Check sheet for the modelled part. Datum: model origin and axes. Units: mm. Coordinates: 2 decimals unless noted, no trailing zeros. Order: outer loops, then holes, each group sorted by start corner. A loop starts at its lowest first (then second) coordinate and runs counter-clockwise, first axis right, second up.
1. Gauge pin test, flat ends, axial feed: pin 1 Ø1 at (y, z) = (-16, 3) entering from +X; pin 2 Ø2.5 at (x, y) = (11.075, -27) entering from -Z; pin 3 Ø1.7 at (x, y) = (15.575, 21.5) entering from +Z. Record the tip position at first contact, or that the pin passes through.
2. Cross-section at C-C (y = -27). Enter the section's corners in (x, z) (3 decimals), then the cut area to 3 significant figures.
3. Thickness scan on line 1 (Y direction, x = -8.94, z = 2.9); line 2 (Y direction, x = -8.94, z = 1.95); line 3 (Y direction, x = -9.5, z = 3.3). Record the ranges inside material, lowest first.
4. Cross-section at D-D (y = -10). Enter the section's corners in (x, z) (3 decimals), then the cut area to 3 significant figures.
5. Cross-section at B-B (x = 0). Enter the section's corners in (y, z).
6. Cross-section at A-A (z = 3.4). Enter the section's corners in (x, y), then the cut area to 3 significant figures.
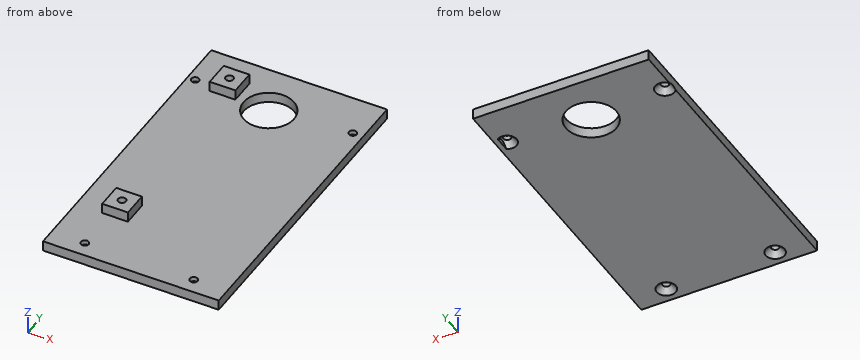
```python
from build123d import *

# Parameters (mm, degrees)
SKETCH1_W           = 33.15
SKETCH1_H           = 60
SKETCH1_R           = 4.9
BOSS_EXTRUDE1_DEPTH = 2
SKETCH3_W           = 5
SKETCH3_H           = 5
BOSS_EXTRUDE2_DEPTH = 2
SKETCH4_R           = 0.75
CUT_EXTRUDE1_DEPTH  = 2
CHAMFER1_SIZE       = 1.1
SKETCH5_W           = 2
SKETCH5_H           = 60
BOSS_EXTRUDE3_DEPTH = 1
SKETCH7_R           = 0.762
CUT_EXTRUDE2_DEPTH  = 3.5


with BuildPart() as part:
    # Sketch1 → Boss-Extrude1 (new body)
    with BuildSketch(Plane.XY):
        Rectangle(SKETCH1_W, SKETCH1_H)
        with Locations((0, 20.1)):
            Circle(SKETCH1_R, mode=Mode.SUBTRACT)
    extrude(amount=BOSS_EXTRUDE1_DEPTH)

    # Sketch3 → Boss-Extrude2 (add)
    with BuildSketch(Plane.XY.offset(2)):
        with Locations((-8.94, 22.5)):
            Rectangle(SKETCH3_W, SKETCH3_H)
        with Locations((-8.94, -15.82)):
            Rectangle(SKETCH3_W, SKETCH3_H)
    extrude(amount=BOSS_EXTRUDE2_DEPTH)

    # Sketch4 → Cut-Extrude1 (cut)
    with BuildSketch(Plane(origin=(0, 0, 0), x_dir=(-1, 0, 0), z_dir=(0, 0, -1))):
        with Locations((-15.575, 21.5)):
            Circle(SKETCH4_R)
        with Locations((15.075, 21.5)):
            Circle(SKETCH4_R)
        with Locations((10.075, -27)):
            Circle(SKETCH4_R)
        with Locations((-11.075, -27)):
            Circle(SKETCH4_R)
    extrude(amount=-CUT_EXTRUDE1_DEPTH, mode=Mode.SUBTRACT)

    # Chamfer1
    # the kernel refuses this chamfer: 1.1 mm, written as the material it takes off along each edge
    with BuildSketch(Plane(origin=(15.575, 21.5, 0), x_dir=(-1, 0, 0), z_dir=(0, -1, 0))) as chamfer1_piece_1:
        Polygon((0.75 + CHAMFER1_SIZE, 0), (0.75, -CHAMFER1_SIZE), (0.75, 0), align=None)
    revolve(axis=Axis((15.575, 21.5, 0), (0, 0, -1)), mode=Mode.SUBTRACT)
    with BuildSketch(Plane(origin=(-15.075, 21.5, 0), x_dir=(-1, 0, 0), z_dir=(0, -1, 0))) as chamfer1_piece_2:
        Polygon((0.75 + CHAMFER1_SIZE, 0), (0.75, -CHAMFER1_SIZE), (0.75, 0), align=None)
    revolve(axis=Axis((-15.075, 21.5, 0), (0, 0, -1)), mode=Mode.SUBTRACT)
    with BuildSketch(Plane(origin=(-10.075, -27, 0), x_dir=(-1, 0, 0), z_dir=(0, -1, 0))) as chamfer1_piece_3:
        Polygon((0.75 + CHAMFER1_SIZE, 0), (0.75, -CHAMFER1_SIZE), (0.75, 0), align=None)
    revolve(axis=Axis((-10.075, -27, 0), (0, 0, -1)), mode=Mode.SUBTRACT)
    with BuildSketch(Plane(origin=(11.075, -27, 0), x_dir=(-1, 0, 0), z_dir=(0, -1, 0))) as chamfer1_piece_4:
        Polygon((0.75 + CHAMFER1_SIZE, 0), (0.75, -CHAMFER1_SIZE), (0.75, 0), align=None)
    revolve(axis=Axis((11.075, -27, 0), (0, 0, -1)), mode=Mode.SUBTRACT)

    # Sketch5 → Boss-Extrude3 (add)
    with BuildSketch(Plane(origin=(16.575, 0, 0), x_dir=(0, 0, -1), z_dir=(1, 0, 0))):
        with Locations((-1, 0)):
            Rectangle(SKETCH5_W, SKETCH5_H)
    extrude(amount=BOSS_EXTRUDE3_DEPTH)

    # Sketch7 → Cut-Extrude2 (cut)
    with BuildSketch(Plane.XY.offset(4)):
        with Locations((-8.94, 22.5)):
            Circle(SKETCH7_R)
        with Locations((-8.94, -15.82)):
            Circle(SKETCH7_R)
    extrude(amount=-CUT_EXTRUDE2_DEPTH, mode=Mode.SUBTRACT)


solid = part.part
```
Data:
1. pin 1: stops at x = -6.44
1. pin 2: stops at z = 0.6
1. pin 3: stops at z = 2
2. outline: (-16.575, 0) - (-11.925, 0) - (-10.825, 1.1) - (-10.825, 2) - (-16.575, 2) - close; (-9.325, 1.1) - (-8.225, 0) - (9.225, 0) - (10.325, 1.1) - (10.325, 2) - (-9.325, 2) - close; (11.825, 1.1) - (12.925, 0) - (17.575, 0) - (17.575, 2) - (11.825, 2) - close
2. area: 59.9 mm2
3. line 1: y = -18.32 to -16.58, -15.06 to -13.32, 20 to 21.74, 23.26 to 25
3. line 2: y = -30 to -16.58, -15.06 to 21.74, 23.26 to 30
3. line 3: y = -18.32 to -16.34, -15.3 to -13.32, 20 to 21.98, 23.02 to 25
4. outline: (-16.575, 0) - (17.575, 0) - (17.575, 2) - (-16.575, 2) - close
4. area: 68.3 mm2
5. outline: (-30, 0) - (15.2, 0) - (15.2, 2) - (-30, 2) - close; (25, 0) - (30, 0) - (30, 2) - (25, 2) - close
6. outline: (-11.44, -18.32) - (-6.44, -18.32) - (-6.44, -13.32) - (-11.44, -13.32) - close; (-11.44, 20) - (-6.44, 20) - (-6.44, 25) - (-11.44, 25) - close; hole circle Ø1.52 at (-8.94, -15.82); hole circle Ø1.52 at (-8.94, 22.5)
6. area: 46.4 mm2
